Geometry check sheet. Reference: drawing and pictorial views, mm from the part's lowest x, y, z. Give positions to 0.01 mm unless a question says otherwise; leave off trailing zeros. Order: outer loops, then holes, each group sorted by start corner. A loop starts at its lowest first (then second) coordinate and runs counter-clockwise, first axis right, second up.
Item 1: Sectioned sample at A-A on y = 40. Record the boundary of the cut face in (x, z), and give its area (3 significant figures).
Item 2: Sectioned sample at C-C on z = 7.75. Record the boundary of the cut face in (x, y).
Item 3: Sectioned sample at B-B on y = 240. Record the boundary of the cut face in (x, z).
Item 4: Sectioned sample at D-D on x = 145. Record the boundary of the cut face in (y, z), and give its area (4 significant figures).
Item 5: Gauge pin test, flat ends, axial feed: P1, Ø13, axis at x = 80, y = 160, coming from the +Z side; P2, Ø4, axis at y = 195.5, z = 2, coming from the -X side. Record the tip position at first contact, or that the pin passes through.
Item 6: Material ranges on line 1 along Y through (x, z) = (80, 8); line 2 along Y through (x, z) = (119, 6); line 3 along Y through (x, z) = (87, 8.5), recorded low to high.
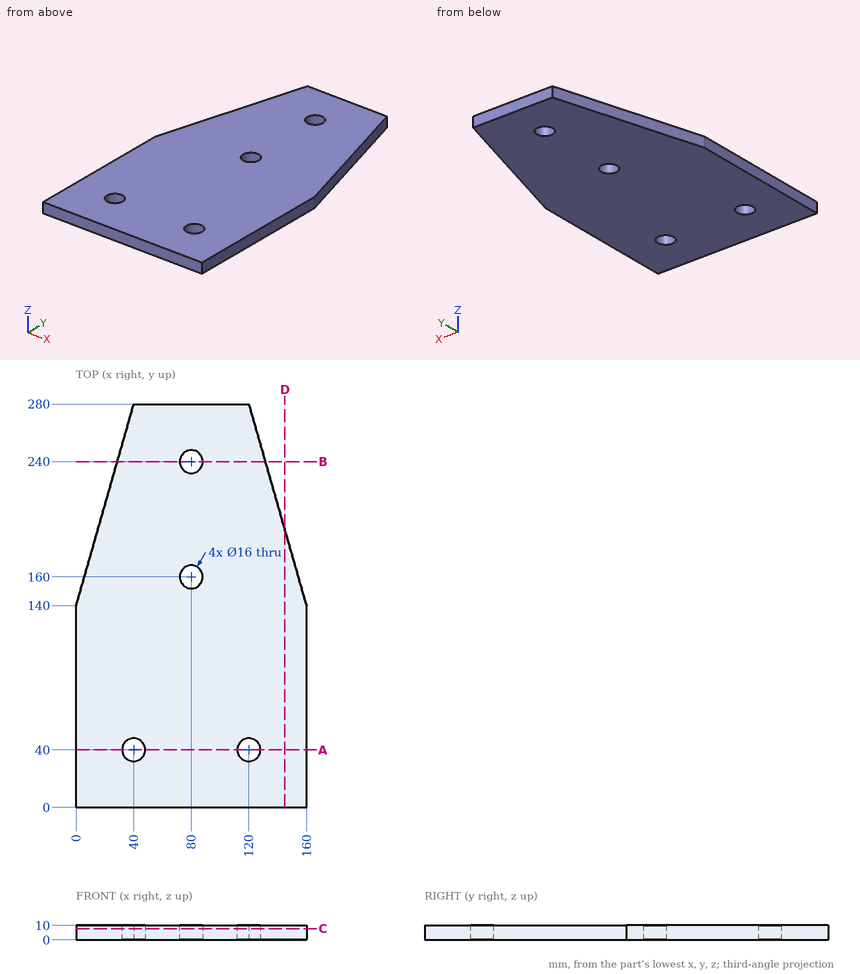
Report:
1. outline: (0, 0) - (32, 0) - (32, 10) - (0, 10) - close; (48, 0) - (112, 0) - (112, 10) - (48, 10) - close; (128, 0) - (160, 0) - (160, 10) - (128, 10) - close
1. area: 1,280 mm2
2. outline: (0, 0) - (160, 0) - (160, 140) - (120, 280) - (40, 280) - (0, 140) - close; hole circle Ø16 at (40, 40); hole circle Ø16 at (80, 160); hole circle Ø16 at (80, 240); hole circle Ø16 at (120, 40)
3. outline: (28.57, 0) - (72, 0) - (72, 10) - (28.57, 10) - close; (88, 0) - (131.43, 0) - (131.43, 10) - (88, 10) - close
4. outline: (0, 0) - (192.5, 0) - (192.5, 10) - (0, 10) - close
4. area: 1,925 mm2
5. P1: passes through
5. P2: stops at x = 15.29
6. line 1: y = 0 to 152, 168 to 232, 248 to 280
6. line 2: y = 0 to 32.06, 47.94 to 280
6. line 3: y = 0 to 156.13, 163.87 to 236.13, 243.87 to 280
